The figure shows three views and two pictorial views of one solid part (mm, origin at its lowest corner). Answer the questions. A direction names the side the tool comes from. Round coordinates to 2 decimals unless told otherwise and drop trailing zeros. Order: outer loops, then holes, each group sorted by start corner. A loop starts at its lowest first (then second) coordinate and runs counter-clockwise, first axis right, second up. Notation, with made-up numbers: (22, -28) - (33, -28) arc R9 ccw to (33, -17) - close; hole circle Ø3 at (34, 30). An arc over 180 degrees is marked (long way). One line per question, with ' | ' between items. Start each with the question number.
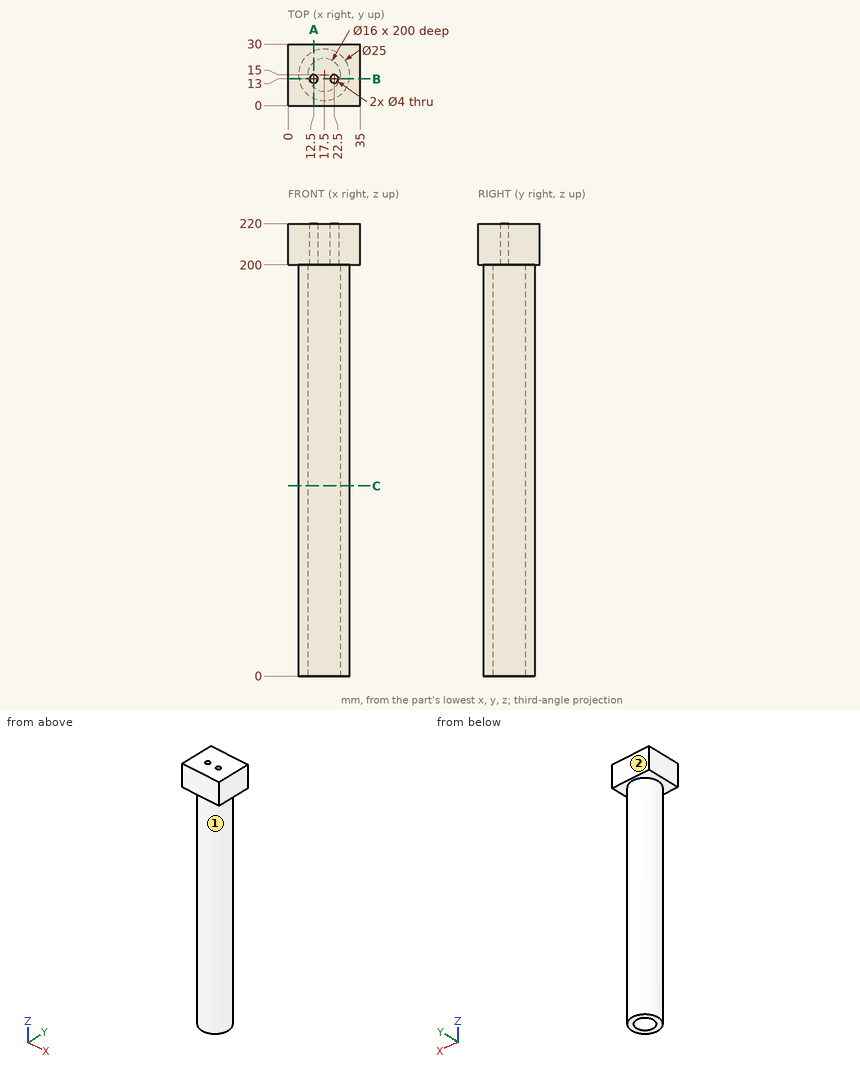
1) For the marked faces 1 and 2, determine the directions among +Z, -Z, +X, -X, +Y, -Y from which every point of the face is accessible in a straight line to the end or side of a thin tool.
2) Section C-C on z = 92.5 is taken. Give the vertices of the cut face in (x, y), and give its area (3 significant figures).
3) Section A-A on x = 12.5 is taken. Give the vertices of the cut face in (y, z) (3 decimals), and give its area (3 significant figures).
4) Section B-B on y = 13 is taken. Give the vertices of the cut face in (x, z), and give its area (3 significant figures).
5) Straight lines are drawn through the part: line 1 (Y direction, x = 12.5, z = 211); line 2 (X direction, y = 14.25, z = 126); line 3 (Y direction, x = 17.5, z = 117). For each, find the intervals that lie inside material, in ascending order.
6) Flat-ended cylindrical pins translate along their axes: pin 1 (8 mm diameter, centred on x = 7, y = 9, fed in from -Z); pin 2 (4 mm diameter, centred on y = 13, z = 61.5, fed in from -X); pin 3 (3 mm diameter, centred on x = 12.5, y = 13, fed in from -Z); pin 4 (5 mm diameter, centred on x = 16.5, z = 169, fed in from -Y). Find the tip coordinate at first contact, or state that the pin passes through.
Recorded:
1) face 1: -Z | face 2: +Z, -Z, +X, -X, +Y
2) outline: circle Ø25 at (17.5, 15); hole circle Ø16 at (17.5, 15) | area: 290 mm²
3) outline: (0, 200) - (3.544, 200) - (3.544, 0) - (8.755, 0) - (8.755, 200) - (11, 200) - (11, 220) - (0, 220) - close; (15, 200) - (21.245, 200) - (21.245, 0) - (26.456, 0) - (26.456, 200) - (30, 200) - (30, 220) - (15, 220) - close | area: 2,600 mm²
4) outline: (0, 200) - (5.16, 200) - (5.16, 0) - (9.75, 0) - (9.75, 200) - (10.5, 200) - (10.5, 220) - (0, 220) - close; (14.5, 200) - (20.5, 200) - (20.5, 220) - (14.5, 220) - close; (24.5, 200) - (25.25, 200) - (25.25, 0) - (29.84, 0) - (29.84, 200) - (35, 200) - (35, 220) - (24.5, 220) - close | area: 2,380 mm²
5) line 1: y = 0 to 11, 15 to 30 | line 2: x = 5.02 to 9.54, 25.46 to 29.98 | line 3: y = 2.5 to 7, 23 to 27.5
6) pin 1: stops at z = 0 | pin 2: stops at x = 5 | pin 3: passes through | pin 4: stops at y = 2.5
